Geometry: final body of the model. Coordinates: model frame, mm. Face numbers are marked on the shaded views. A direction names the side the tool comes from. Round coordinates to 2 decimals unless told otherwise and drop trailing zeros. Write each loop counter-clockwise with the first axis right and the second up, starting at its lowest first coordinate (ties: lowest second). Pieces come first, ordered by that corner, then holes. Notation, with made-up numbers: (88.25, 7.5) - (137.25, 7.5) arc R23 ccw to (137.25, 29.5) - close; hole circle Ø3 at (17, -19). An arc over 180 degrees is marked (long way). Use a Markdown table: item, result. Add a question column.
```python
from build123d import *

# Parameters (mm, degrees)
SKETCH1_W           = 50
SKETCH1_H           = 60
SKETCH1_W_2         = 47
SKETCH1_H_2         = 57
BOSS_EXTRUDE6_DEPTH = 40
SKETCH7_W           = 50
SKETCH7_H           = 60
BOSS_EXTRUDE8_DEPTH = 1.5
SKETCH8_W           = 10
SKETCH8_H           = 2
BOSS_EXTRUDE9_DEPTH = 50
SKETCH9_R           = 1.55
CUT_EXTRUDE1_DEPTH  = 3
SKETCH11_R          = 8.25
CUT_EXTRUDE3_DEPTH  = 1.5


with BuildPart() as part:
    # Sketch1 → Boss-Extrude6 (new body)
    with BuildSketch(Plane(origin=(0, 0, 0), x_dir=(1, 0, 0), z_dir=(0, 1, 0))):
        Rectangle(SKETCH1_W, SKETCH1_H)
        Rectangle(SKETCH1_W_2, SKETCH1_H_2, mode=Mode.SUBTRACT)
    extrude(amount=BOSS_EXTRUDE6_DEPTH)

    # Sketch7 → Boss-Extrude8 (add)
    with BuildSketch(Plane.XZ):
        Rectangle(SKETCH7_W, SKETCH7_H)
    extrude(amount=BOSS_EXTRUDE8_DEPTH)

    # Sketch8 → Boss-Extrude9 (add)
    with BuildSketch(Plane(origin=(25, 0, 0), x_dir=(0, 0, -1), z_dir=(1, 0, 0))):
        with Locations((-35, 39)):
            Rectangle(SKETCH8_W, SKETCH8_H)
        with Locations((35, 39)):
            Rectangle(SKETCH8_W, SKETCH8_H)
    extrude(amount=-BOSS_EXTRUDE9_DEPTH)

    # Sketch9 → Cut-Extrude1 (cut)
    with BuildSketch(Plane(origin=(0, 40, 0), x_dir=(1, 0, 0), z_dir=(0, 1, 0))):
        with Locations(Location((-20, 35, 0), (0, 0, 270))):
            Circle(SKETCH9_R)
        with Locations(Location((20, 35, 0), (0, 0, 270))):
            Circle(SKETCH9_R)
        with Locations(Location((20, -35, 0), (0, 0, 270))):
            Circle(SKETCH9_R)
        with Locations(Location((-20, -35, 0), (0, 0, 270))):
            Circle(SKETCH9_R)
    extrude(amount=-CUT_EXTRUDE1_DEPTH, mode=Mode.SUBTRACT)

    # Sketch11 → Cut-Extrude3 (cut)
    with BuildSketch(Plane.ZY.offset(25)):
        with Locations((0, 18.25)):
            Circle(SKETCH11_R)
    extrude(amount=-CUT_EXTRUDE3_DEPTH, mode=Mode.SUBTRACT)


solid = part.part
```
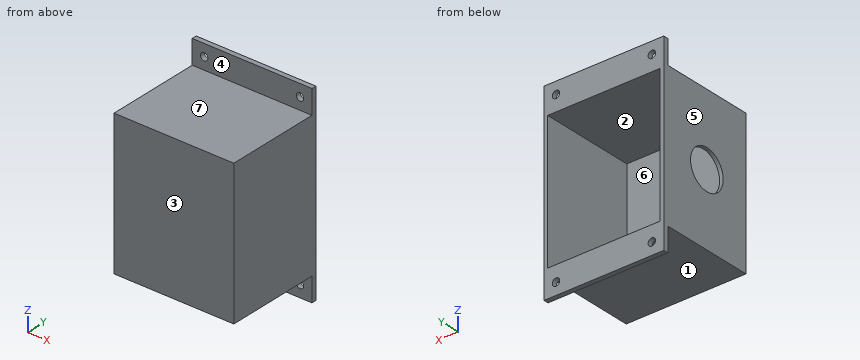
1) Set-up query: the marked faces 1, 2, 3 and 4. Return all of +Z, -Z, +X, -X, +Y, -Y with unobstructed straight access to the full face (end or side cutting, diameter ignored); none if empty.
2) Section B-B, the plane y = 32. Return the cut outline in (x, z).
3) Pin query (flat end, axial travel): P1, Ø5, axis at x = -8.5, y = 8.5, coming from the +Z side; P2, Ø2, axis at x = -14.5, z = 11, coming from the +Y side; P3, Ø1.9, axis at x = -20, z = -35, coming from the +Y side; P4, Ø12, axis at x = -5.5, y = 25, coming from the -Z side. Return the tip coordinate at first contact, or that it passes through.
4) Draft query along Z for the marked faces 5, 6 and 7. Return one class per face: released by +Z, released by -Z, zero draft, split by the parting line, or undercut.
5) Section D-D, the plane z = -25. Return the cut outline in (x, y).
6) Material intervals for L1, parallel to X at y = 39.2, z = -35; L2, parallel to Z at x = -2, y = 24; L3, parallel to X at y = 6.5, z = 7, sorted ascending. Write a range as from..to.
7) Section C-C, the plane z = -35. Return the cut outline in (x, y).
8) Section A-A, the plane x = 20. Return the cut outline in (y, z).
Output values:
| question | item | result |
|---|---|---|
| 1 | face 1 | -Z, +X, -X, -Y |
| 1 | face 2 | +Y |
| 1 | face 3 | +Z, -Z, +X, -X, -Y |
| 1 | face 4 | +Z, +X, -X, -Y |
| 2 | outline | (-25, -30) - (25, -30) - (25, 30) - (-25, 30) - close; hole (-23.5, -28.5) - (23.5, -28.5) - (23.5, 28.5) - (-23.5, 28.5) - close |
| 3 | P1 | stops at z = 30 |
| 3 | P2 | stops at y = 0 |
| 3 | P3 | passes through |
| 3 | P4 | stops at z = -30 |
| 4 | face 5 | zero draft |
| 4 | face 6 | undercut |
| 4 | face 7 | released by +Z |
| 5 | outline | (-25, -1.5) - (25, -1.5) - (25, 40) - (23.5, 40) - (23.5, 0) - (-23.5, 0) - (-23.5, 40) - (-25, 40) - close |
| 6 | L1 | x = -25..-21.55, -18.45..18.45, 21.55..25 |
| 6 | L2 | z = -30..-28.5, 28.5..30 |
| 6 | L3 | x = -25..-23.5, 23.5..25 |
| 7 | outline | (-25, 38) - (-21.55, 38) - (-21.55, 40) - (-25, 40) - close; (-18.45, 38) - (18.45, 38) - (18.45, 40) - (-18.45, 40) - close; (21.55, 38) - (25, 38) - (25, 40) - (21.55, 40) - close |
| 8 | outline | (-1.5, -30) - (38, -30) - (38, -33.45) - (40, -33.45) - (40, -28.5) - (0, -28.5) - (0, 28.5) - (40, 28.5) - (40, 33.45) - (38, 33.45) - (38, 30) - (-1.5, 30) - close; (38, -40) - (40, -40) - (40, -36.55) - (38, -36.55) - close; (38, 36.55) - (40, 36.55) - (40, 40) - (38, 40) - close |
